from build123d import *

# Parameters (mm, degrees)
EXTRUDE_1_DEPTH     = 50
EXTRUDE_2_DEPTH     = 2
EXTRUDE_4_DEPTH     = 2
SKETCH_4_R          = 13
SKETCH_4_R_2        = 2
CUT_EXTRUDE_1_DEPTH = 3
SKETCH_5_R          = 12.5
SKETCH_5_R_2        = 2.5
CUT_EXTRUDE_2_DEPTH = 3
FILLET_2_R          = 2


with BuildPart() as part:
    # 草图1 → 凸台-拉伸1 (new body)
    with BuildSketch(Plane(origin=(0, 0, 0), x_dir=(0, 0, -1), z_dir=(1, 0, 0))):
        Polygon((0, 0), (0, 50), (-2, 50), (-2, 2), (-50, 2), (-50, 0), align=None)
    extrude(amount=EXTRUDE_1_DEPTH)

    # 草图2 → 凸台-拉伸2 (add)
    with BuildSketch(Plane(origin=(50, 0, 0), x_dir=(0, 0, -1), z_dir=(1, 0, 0))):
        Polygon((-2, 26), (-26, 2), (-2, 2), align=None)
    extrude(amount=-EXTRUDE_2_DEPTH)

    # 草图3 → 凸台-拉伸4 (add)
    with BuildSketch(Plane.ZY):
        Polygon((2, 26), (26, 2), (2, 2), align=None)
    extrude(amount=-EXTRUDE_4_DEPTH)

    # 草图4 → 切除-拉伸1 (cut, through all)
    with BuildSketch(Plane.XY.offset(2)):
        with Locations((25, 28)):
            Circle(SKETCH_4_R)
        with Locations((25, 45.5)):
            Circle(SKETCH_4_R_2)
        with Locations((42.5, 28)):
            Circle(SKETCH_4_R_2)
        with Locations((25, 10.5)):
            Circle(SKETCH_4_R_2)
        with Locations((7.5, 28)):
            Circle(SKETCH_4_R_2)
    extrude(amount=-CUT_EXTRUDE_1_DEPTH, mode=Mode.SUBTRACT)

    # 草图5 → 切除-拉伸2 (cut, through all)
    with BuildSketch(Plane(origin=(0, 2, 0), x_dir=(1, 0, 0), z_dir=(0, 1, 0))):
        with Locations((25, -26)):
            Circle(SKETCH_5_R)
        with Locations((10, -11)):
            Circle(SKETCH_5_R_2)
        with Locations((40, -11)):
            Circle(SKETCH_5_R_2)
        with Locations((40, -41)):
            Circle(SKETCH_5_R_2)
        with Locations((10, -41)):
            Circle(SKETCH_5_R_2)
    extrude(amount=-CUT_EXTRUDE_2_DEPTH, mode=Mode.SUBTRACT)

    # 圆角2
    fillet_2_edges = [part.edges().sort_by_distance(p)[0] for p in [
        (25, 0, 0),
    ]]
    fillet(fillet_2_edges, radius=FILLET_2_R)


solid = part.part
The model under review builds one solid part; all positions refer to its coordinate system, in mm. A direction names the side the tool comes from. Round coordinates to 2 decimals unless told otherwise and drop trailing zeros. Write each loop counter-clockwise with the first axis right and the second up, starting at its lowest first coordinate (ties: lowest second). Pieces come first, ordered by that corner, then holes. Notation, with made-up numbers: (0, 63) - (40, 63) arc R28 ccw to (40, 87) - close; hole circle Ø3 at (57, 66). An arc over 180 degrees is marked (long way). One line per item, written item: value. Start each with the question number.
1. Clearance check with flat-ended pins moving along their axes: P1, Ø6, axis at x = 10, z = 24, coming from the -Y side; P2, Ø1.5, axis at x = 11.5, y = 36, coming from the +Z side; P3, Ø12, axis at x = 20, z = 31, coming from the +Y side. State where each tip first meets the part, or that it passes through.
2. Consider section D-D on z = 20.5. Write out the cut boundary in (x, y), and give its area (3 significant figures).
3. The part is to be moulded in two halves that separate along Y. For faces 3 (the face through (7.066, 26.048, 1.014)), 4 (the face through (9.46, 1.01, 43.44)), 5 (the face through (42.066, 26.048, 1.014)), 6 (the face through (49, 14, 14)), say which applies: released by +Y, released by -Y, zero draft, split by the parting line, or undercut.
4. To check wall thickness, follow L1, parallel to Z at x = 40, y = 1; L2, parallel to X at y = 0.75, z = 26; L3, parallel to Y at x = 3, z = 24. State the ranges of each line that lie inside material, in increasing order. Write a range as from..to.
5. Consider section A-A on y = 45.5. Write out the cut boundary in (x, z), and give its area (3 significant figures).
6. Machinability: for faces 1 (the face through (25.35, 0.57, 0.6)), 2 (the face through (13.5, 2, 20.3)), which of the approach directions +Z, -Z, +X, -X, +Y, -Y give a long, thin tool a straight path to every point of the face, cutting with its end or side? Answer none if there is none.
7. Consider section B-B on z = 11. Write out the cut boundary in (x, y), and give its area (3 significant figures).
8. Consider section C-C on x = 24.5. Write out the cut boundary in (y, z), and give its area (3 significant figures).
Checks:
1. P1: stops at y = 0
1. P2: stops at z = 2
1. P3: stops at y = 2
2. outline: (0, 0) - (13.78, 0) - (13.78, 2) - (2, 2) - (2, 7.5) - (0, 7.5) - close; (36.22, 0) - (50, 0) - (50, 7.5) - (48, 7.5) - (48, 2) - (36.22, 2) - close
2. area: 77.1 mm^2
3. face 3: undercut
3. face 4: zero draft
3. face 5: undercut
3. face 6: released by +Y
4. L1: z = 0.27..8.5, 13.5..38.5, 43.5..50
4. L2: x = 0..12.5, 37.5..50
4. L3: y = 0..2
5. outline: (0, 0) - (23, 0) - (23, 2) - (0, 2) - close; (27, 0) - (50, 0) - (50, 2) - (27, 2) - close
5. area: 92.0 mm^2
6. face 1: -Z, +X, -X, -Y
6. face 2: +Z, +Y
7. outline: (0, 0) - (7.5, 0) - (7.5, 2) - (2, 2) - (2, 17) - (0, 17) - close; (12.5, 0) - (37.5, 0) - (37.5, 2) - (12.5, 2) - close; (42.5, 0) - (50, 0) - (50, 17) - (48, 17) - (48, 2) - (42.5, 2) - close
7. area: 140 mm^2
8. outline: (0, 2) arc R2 ccw to (2, 0) - (8.56, 0) - (8.56, 2) - (2, 2) - (2, 13.51) - (0, 13.51) - close; (0, 38.49) - (2, 38.49) - (2, 50) - (0, 50) - close; (12.44, 0) - (15.01, 0) - (15.01, 2) - (12.44, 2) - close; (40.99, 0) - (43.56, 0) - (43.56, 2) - (40.99, 2) - close; (47.44, 0) - (50, 0) - (50, 2) - (47.44, 2) - close
8. area: 77.7 mm^2
